```python
from build123d import *

# Parameters (mm, degrees)
SKETCH2_R               = 15
CUT_EXTRUDE1_DEPTH      = 16
CUT_EXTRUDE1_DEPTH_BACK = 16
SKETCH3_W               = 17.5
SKETCH3_H               = 7
CUT_EXTRUDE2_DEPTH      = 16
CUT_EXTRUDE2_DEPTH_BACK = 16


with BuildPart() as part:
    # Sketch1 → Revolve1 (revolve)
    with BuildSketch(Plane.XY):
        Polygon((12.5, 75), (8.480762114, 60), (2.5, 60), (2.5, 26.655097241), (15, 26), (15, 0), (-15, 0), (-15, 26), (-2.5, 26.655097241), (-2.5, 60), (-8.480762114, 60), (-12.5, 75), (-7.323619098, 75), (-4.644127174, 65), (4.644127174, 65), (7.323619098, 75), align=None)
    revolve(axis=Axis((15, 0, 0), (-1, 0, 0)))

    # Sketch2 → Cut-Extrude1 (cut, two sides)
    with BuildSketch(Plane(origin=(0, 0, 0), x_dir=(0, 0, -1), z_dir=(1, 0, 0))) as cut_extrude1_sk:
        Circle(SKETCH2_R)
    extrude(amount=CUT_EXTRUDE1_DEPTH, mode=Mode.SUBTRACT)
    extrude(cut_extrude1_sk.sketch, amount=-CUT_EXTRUDE1_DEPTH_BACK, mode=Mode.SUBTRACT)

    # Sketch3 → Cut-Extrude2 (cut, two sides)
    with BuildSketch(Plane(origin=(0, 0, 0), x_dir=(0, 0, -1), z_dir=(1, 0, 0))) as cut_extrude2_sk:
        with Locations((-8.75, 0)):
            Rectangle(SKETCH3_W, SKETCH3_H)
    extrude(amount=CUT_EXTRUDE2_DEPTH, mode=Mode.SUBTRACT)
    extrude(cut_extrude2_sk.sketch, amount=-CUT_EXTRUDE2_DEPTH_BACK, mode=Mode.SUBTRACT)


solid = part.part
```
For this review, take the finished solid that the model builds, in its own axes (mm). A direction names the side the tool comes from. Round coordinates to 2 decimals unless told otherwise and drop trailing zeros. Answer as CSV lines item,"result". Start each with the question number.
(1) For pin 1 (5 mm diameter, centred on y = -25.5, z = 39, fed in from +X); pin 2 (3 mm diameter, centred on x = 9, z = 16, fed in from +Y) (3 decimals); pin 3 (6 mm diameter, centred on x = 4.5, y = -7, fed in from +Z), all flat-tipped, find the tip position at first contact; note any pin that passes through.
(2) Mouldability with a two-part tool opening along Y and no side actions: class faces 5 (the flat face through (-15, -11, 11)), 6 (the conical face through (-8.732, -13.21, 59.489)), 7 (the conical face through (-4.774, 62.462, -19.67)) as +Y half, -Y half, draft (parallel to the pull), parting line (faces both ways), or undercut.
(3) Machinability: for faces 1 (the flat face through (0, 0, 17.5)), 2 (the cylindrical face through (-5.53, -59.94, -2.64)), 3 (the cylindrical face through (0.07, 62, -19.52)), 4 (the cylindrical face through (5.45, -59.94, -2.64)), which of the approach directions +Z, -Z, +X, -X, +Y, -Y give a long, thin tool a straight path to every point of the face, cutting with its end or side? Answer none if there is none.
(4) For line 1 (X direction, y = 37, z = 4.5); line 2 (Y direction, x = 4.35, z = 0); line 3 (Z direction, x = 0.5, y = -12.5), list the stretches that pass through material, from the lowest coordinate up.
From the geometry:
1,pin 1,"stops at x = 2.5"
1,pin 2,"stops at y = 73.585"
1,pin 3,"stops at z = 74.76"
2,face 5,"draft"
2,face 6,"undercut"
2,face 7,"parting line"
3,face 1,"+X, -X"
3,face 2,"-X"
3,face 3,"none"
3,face 4,"+X"
4,line 1,"x = -2.5 to 2.5"
4,line 2,"y = -65 to -60, -26.56 to -15, 15 to 26.56, 60 to 65"
4,line 3,"z = -63.79 to -8.29, 8.29 to 63.79"
